from build123d import *

# Parameters (mm, degrees)
F0_W      = 38
F0_H      = 38
F1_DEPTH  = 15
F2_R      = 12.9
F3_DEPTH  = 28
F4_R      = 3.4
F5_DEPTH  = 21
F7_DEPTH  = 38
F8_R      = 14
F9_DEPTH  = 65
F10_R     = 16.05
F11_DEPTH = 30
F12_W     = 50
F12_H     = 50
F12_R     = 16.05
F13_DEPTH = 30
F14_R     = 9
F15_DEPTH = 109.2397803647
F16_R     = 1.2
F17_DEPTH = 115.2397803647
F18_R     = 1.2
F19_DEPTH = 50.001
F20_SIZE  = 5
F21_SIZE  = 1


with BuildPart() as f1:
    # F0 (on Top) → F1 (new body)
    with BuildSketch(Plane.XY):
        Rectangle(F0_W, F0_H)
    extrude(amount=F1_DEPTH)

    # F2 (on face) → F3 (join)
    with BuildSketch(Plane(origin=(0, 0, 0), x_dir=(1, 0, 0), z_dir=(0, 0, -1))):
        Circle(F2_R)
    extrude(amount=F3_DEPTH)

    # F4 (on Front) → F5 (cut, symmetric)
    with BuildSketch(Plane.XZ):
        with Locations((0, -15)):
            Circle(F4_R)
    extrude(amount=F5_DEPTH, both=True, mode=Mode.SUBTRACT)

    # F6 (on face) → F7 (join)
    with BuildSketch(Plane.YZ.offset(19)):
        Polygon((-71.4847223192, 75.3767664178), (-19, 15), (19, 15), (19, 29.2076178204), (-42.8057582708, 100.3070095195), align=None)
    extrude(amount=-F7_DEPTH)

    # F8 (on face) → F9 (cut)
    with BuildSketch(Plane(origin=(0, -68.0895883757, 78.3281113281), x_dir=(1, 0, 0), z_dir=(0, -0.656059029, 0.7547095802))):
        with Locations((0, 14.5014034106)):
            Circle(F8_R)
    extrude(amount=-F9_DEPTH, mode=Mode.SUBTRACT)

    # F10 (on face) → F11 (cut)
    with BuildSketch(Plane(origin=(0, -68.0895883757, 78.3281113281), x_dir=(1, 0, 0), z_dir=(0, -0.656059029, 0.7547095802))):
        with Locations((0, 14.5014034106)):
            Circle(F10_R)
    extrude(amount=-F11_DEPTH, mode=Mode.SUBTRACT)

    # F12 (on face) → F13 (join)
    with BuildSketch(Plane(origin=(0, -68.0895883757, 78.3281113281), x_dir=(1, 0, 0), z_dir=(0, -0.656059029, 0.7547095802))):
        with Locations((0, 14.5014034106)):
            Rectangle(F12_W, F12_H)
        with Locations((0, 14.5014034106)):
            Circle(F12_R, mode=Mode.SUBTRACT)
    extrude(amount=-F13_DEPTH)

    # F14 (on face) → F15 (cut, through all)
    with BuildSketch(Plane(origin=(0, 25.2838301049, 21.9788981914), x_dir=(-1, 0, 0), z_dir=(0, 0.7547095802, 0.656059029))):
        with Locations((0, 48.7857652542)):
            Circle(F14_R)
    extrude(amount=-F15_DEPTH, mode=Mode.SUBTRACT)

    # F16 (on face) → F17 (cut, through all)
    with BuildSketch(Plane(origin=(0, 29.8120875862, 25.9152523653), x_dir=(-1, 0, 0), z_dir=(0, 0.7547095802, 0.656059029))):
        with Locations((0, 95.7857652542)):
            Circle(F16_R)
        with Locations((0, 81.7857652542)):
            Circle(F16_R)
    extrude(amount=-F17_DEPTH, mode=Mode.SUBTRACT)

    # F18 (on face) → F19 (cut, through all)
    with BuildSketch(Plane.YZ.offset(25)):
        with Locations((-51.8967680631, 81.8042113269)):
            Circle(F18_R)
        with Locations((-42.7119416572, 71.2382772037)):
            Circle(F18_R)
    extrude(amount=-F19_DEPTH, mode=Mode.SUBTRACT)

    # F20
    f20_edges = [f1.edges().sort_by_distance(p)[0] for p in [
        (-12.9, 0, -28),
        (25, -28.436615, 92.92272),
        (25, -66.172094, 60.119769),
        (-25, -66.172094, 60.119769),
        (-25, -28.436615, 92.92272),
    ]]
    chamfer(f20_edges, length=F20_SIZE)

    # F21
    f21_edges = [f1.edges().sort_by_distance(p)[0] for p in [
        (-16.05, -57.14524, 87.841888),
        (9, -35.401476, 33.86774),
        (9, -6.722512, 58.797983),
    ]]
    chamfer(f21_edges, length=F21_SIZE)


solid = f1.part
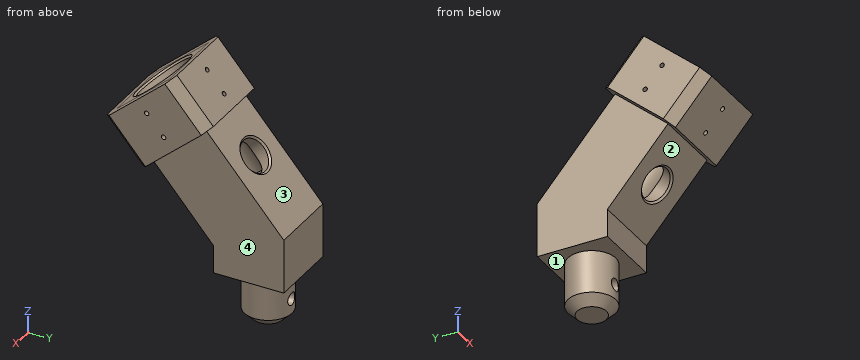
Geometry: final body of the model. Coordinates: model frame, mm. Face numbers are marked on the shaded views. A direction names the side the tool comes from. Coordinates: 2 decimals unless noted, no trailing zeros. Loops run counter-clockwise (first coordinate to the right, second up) from the corner with the lowest first, then second, coordinate; pieces in that order, holes last. Notation, with made-up numbers: M -19,28 L -7,28 A31 ccw -7,67 Z; hole C 5,51.25 d5. An arc over 180 degrees is marked long. One line per item, written item: value. Start each with the question number.
1) Cut plane B-B (z = 17.5). Return loops of the section in (x, y).
2) Cut plane A-A (z = -6). Return loops of the section in (x, y).
3) Reachability of the marked faces 1, 2, 3 and 4 from +Z, -Z, +X, -X, +Y, -Y: full face, straight path, thin tool, end or side. Return the list, or none.
4) Pin query (flat end, axial travel): P1, Ø21, axis at y = -33.5, z = 23, coming from the +X side; P2, Ø3, axis at x = -3.5, y = -1.5, coming from the +Z side; P3, Ø1, axis at y = -50, z = 48, coming from the +X side; P4, Ø12, axis at x = 6.5, z = 8.5, coming from the -Y side. Return the tip coordinate at first contact, or that it passes through.
5) Material intervals for L1, parallel to X at y = -26, z = 52.5; L2, parallel to X at y = 2.5, z = -15; L3, parallel to X at y = -5.5, z = 26, sorted ascending. Write a range as from..to.
Evaluation:
1. outline: M -19,-21.17 L 19,-21.17 L 19,19 L -19,19 Z
2. outline: C 0,0 d25.8
3. face 1: -Z
3. face 2: -Z, +X, -X
3. face 3: +X, -X, +Y
3. face 4: -Z, +X, +Y
4. P1: x = 19
4. P2: z = 52.37
4. P3: through
4. P4: y = -19
5. L1: -19..-14, 14..19
5. L2: -12.66..-3.4, 3.4..12.66
5. L3: -19..19
